from build123d import *

# Parameters (mm, degrees)
F0_R     = 60.567537
F1_DEPTH = 25.4
F2_R     = 43.725742
F3_DEPTH = 19.801166
F4_W     = 52.260071
F4_H     = 50.955355
F5_DEPTH = 118.063478


with BuildPart() as f1:
    # F0 (on Front) → F1 (new body)
    with BuildSketch(Plane.XZ):
        Circle(F0_R)
    extrude(amount=F1_DEPTH)

    # F2 (on face) → F3 (join)
    with BuildSketch(Plane.XZ.offset(25.4)):
        Circle(F2_R)
    extrude(amount=F3_DEPTH)

    # F4 (on face) → F5 (cut)
    with BuildSketch(Plane(origin=(0, 0, 0), x_dir=(-1, 0, 0), z_dir=(0, 1, 0))):
        with Locations((5.000293, -0.476226)):
            Rectangle(F4_W, F4_H)
    extrude(amount=-F5_DEPTH, mode=Mode.SUBTRACT)


solid = f1.part
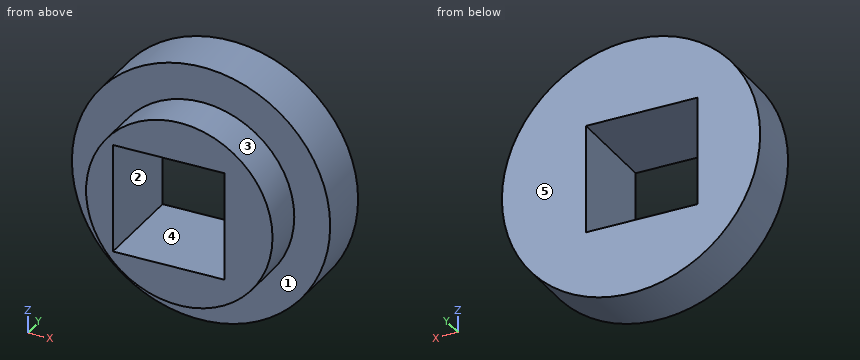
Input: part model. Units: mm. Frame: model coordinates. Face numbers are marked on the shaded views. A direction names the side the tool comes from. Give positions to 0.01 mm unless a question says otherwise; leave off trailing zeros. Loops run counter-clockwise (first coordinate to the right, second up) from the corner with the lowest first, then second, coordinate; pieces in that order, holes last. Notation, with made-up numbers: M 18.5,8 L 27.5,8 A14 cw 27.5,14 Z; hole C 17,-6 d3. An arc over 180 degrees is marked long. Use one line per item in the form item = value.
1. Reachability of the marked faces 4 and 5 from +Z, -Z, +X, -X, +Y, -Y: full face, straight path, thin tool, end or side. Return the list, or none.
Numbers:
face_4 = +Y, -Y
face_5 = +Z, -Z, +X, -X, +Y
2. Line query: L1, parallel to Z at x = 0, y = -9.5; L2, parallel to Y at x = 46, z = 19.5; L3, parallel to Z at x = -20, y = -14. Output: solid intervals per line, ascending.
Numbers:
L1 = -60.57 to -25.95, 25 to 60.57
L2 = -25.4 to 0
L3 = -57.17 to -25.95, 25 to 57.17
3. Section query B-B, the plane z = 0. Return the cut outline in (x, y).
Numbers:
outline = M -60.57,-25.4 L -43.73,-25.4 L -43.73,-45.2 L -31.13,-45.2 L -31.13,0 L -60.57,0 Z; M 21.13,-45.2 L 43.73,-45.2 L 43.73,-25.4 L 60.57,-25.4 L 60.57,0 L 21.13,0 Z
4. Pull-direction query (Z, two-part tool) for the marked faces 1, 2 and 3; classes: released by +Z, released by -Z, zero draft, split by the parting line, or undercut.
Numbers:
face_1 = zero draft
face_2 = undercut
face_3 = split by the parting line
5. Section query A-A, the plane x = 0. Return the cut outline in (y, z).
Numbers:
outline = M -45.2,-43.73 L -25.4,-43.73 L -25.4,-60.57 L 0,-60.57 L 0,-25.95 L -45.2,-25.95 Z; M -45.2,25 L 0,25 L 0,60.57 L -25.4,60.57 L -25.4,43.73 L -45.2,43.73 Z
6. Section query D-D, the plane z = 33.5. Return the cut outline in (x, y).
Numbers:
outline = M -50.46,-25.4 L -28.1,-25.4 L -28.1,-45.2 L 28.1,-45.2 L 28.1,-25.4 L 50.46,-25.4 L 50.46,0 L -50.46,0 Z
7. First-contact query: pin 1 (5 mm diameter, centred on x = 9, y = -10, fed in from -Z); pin 2 (5 mm diameter, centred on y = -12.5, z = 30, fed in from -X); pin 3 (5 mm diameter, centred on y = -31, z = -12, fed in from +X). Flat tips, straight axial feed; report the tip coordinate or a pass-through.
Numbers:
pin_1 = -60.22
pin_2 = -53.96
pin_3 = 42.68
8. Section query C-C, the plane y = -21. Return the cut outline in (x, z), and give its area (3 significant figures).
Numbers:
outline = C 0,0 d121.14; hole M -31.13,-25.95 L 21.13,-25.95 L 21.13,25 L -31.13,25 Z
area = 8,860 mm²
